Build history of the part. All positions in model axes, mm. Face numbers are marked on the shaded views. A direction names the side the tool comes from. Give positions to 0.01 mm unless a question says otherwise; leave off trailing zeros. Order: outer loops, then holes, each group sorted by start corner. A loop starts at its lowest first (then second) coordinate and runs counter-clockwise, first axis right, second up. Notation, with made-up numbers: (70, 1) - (98, 1) arc R29 cw to (98, 34) - close; hole circle Ø8 at (89, 20.25). An arc over 180 degrees is marked (long way). One line per item, written item: value.
```python
from build123d import *

# Parameters (mm, degrees)
F0_W        = 20
F0_H        = 50
F0_W_2      = 16
F0_H_2      = 46
F1_DEPTH    = 2
F2_DEPTH    = 36
F4_DEPTH    = 10
F5_R        = 1.875
F6_DEPTH    = 25
F7_T1_DEPTH = 2
F7_T3_DEPTH = 2
F7_T5_DEPTH = 61
F7_T7_DEPTH = 27
F7_T9_DEPTH = 75
F8_DEPTH    = 3
F9_DEPTH    = 3


# Not quite as in the source:
# - a fillet or chamfer that OpenCascade refuses, or shapes differently, is made with other operations: its cross-section is extruded or revolved along the edge and cut away or added


with BuildPart() as f1:
    # F0 (on Top) → F1 (new body)
    with BuildSketch(Plane.XY):
        Rectangle(F0_W, F0_H)
        Rectangle(F0_W_2, F0_H_2, mode=Mode.SUBTRACT)
        Rectangle(F0_W_2, F0_H_2)
    extrude(amount=F1_DEPTH)

    # F0 (on Top) → F2 (join)
    with BuildSketch(Plane.XY):
        Rectangle(F0_W, F0_H)
        Rectangle(F0_W_2, F0_H_2, mode=Mode.SUBTRACT)
    extrude(amount=F2_DEPTH)

    # F3 (on face) → F4 (join)
    with BuildSketch(Plane.XY.offset(36)):
        Polygon((10, -25), (10, 25), (8, 25), (8, 23), (8, -23), (8, -25), align=None)
    extrude(amount=F4_DEPTH)

    # F5 (on face) → F6 (cut)
    with BuildSketch(Plane(origin=(8, 0, 0), x_dir=(0, -1, 0), z_dir=(-1, 0, 0))):
        with Locations((15, 41)):
            Circle(F5_R)
        with Locations((-15, 41)):
            Circle(F5_R)
    extrude(amount=-F6_DEPTH, mode=Mode.SUBTRACT)

    # F7: fillet of radius 5 on 7 edges, made by hand

    # F7_s2 → F7_t1 (join)
    with BuildSketch(Plane.XZ.offset(23)):
        with BuildLine():
            ThreePointArc((8, 41), (6.5355339059, 37.4644660941), (3, 36))
            Line((3, 36), (8, 36))
            Line((8, 36), (8, 41))
        make_face()
    extrude(amount=F7_T1_DEPTH)

    # F7_s4 → F7_t3 (join)
    with BuildSketch(Plane.XZ.offset(-25)):
        with BuildLine():
            ThreePointArc((8, 41), (6.5355339059, 37.4644660941), (3, 36))
            Line((3, 36), (8, 36))
            Line((8, 36), (8, 41))
        make_face()
    extrude(amount=F7_T3_DEPTH)

    # F7_s6 → F7_t5 (cut)
    with BuildSketch(Plane.XY.offset(-12.5)):
        with BuildLine():
            ThreePointArc((-5, -25), (-8.5355339059, -23.5355339059), (-10, -20))
            Line((-10, -20), (-10, -25))
            Line((-10, -25), (-5, -25))
        make_face()
        with BuildLine():
            ThreePointArc((-5, 25), (-8.5355339059, 23.5355339059), (-10, 20))
            Line((-10, 20), (-10, 25))
            Line((-10, 25), (-5, 25))
        make_face()
    extrude(amount=F7_T5_DEPTH, mode=Mode.SUBTRACT)

    # F7_s8 → F7_t7 (cut)
    with BuildSketch(Plane.YZ.offset(-4.5)):
        with BuildLine():
            ThreePointArc((-25, 41), (-23.5355339059, 44.5355339059), (-20, 46))
            Line((-20, 46), (-25, 46))
            Line((-25, 46), (-25, 41))
        make_face()
        with BuildLine():
            ThreePointArc((25, 41), (23.5355339059, 44.5355339059), (20, 46))
            Line((20, 46), (25, 46))
            Line((25, 46), (25, 41))
        make_face()
    extrude(amount=F7_T7_DEPTH, mode=Mode.SUBTRACT)

    # F7_s10 → F7_t9 (cut)
    with BuildSketch(Plane.XZ.offset(-37.5)):
        with BuildLine():
            ThreePointArc((-10, 31), (-8.5355339059, 34.5355339059), (-5, 36))
            Line((-5, 36), (-10, 36))
            Line((-10, 36), (-10, 31))
        make_face()
    extrude(amount=F7_T9_DEPTH, mode=Mode.SUBTRACT)

    # F8 (add): a face of the model
    f8_faces = [f1.faces().sort_by_distance(p)[0] for p in [
        (10, 0, 22.721056124),
    ]]
    extrude(f8_faces, amount=F8_DEPTH)

    # F5 (on face) → F9 (cut)
    with BuildSketch(Plane(origin=(8, 0, 0), x_dir=(0, -1, 0), z_dir=(-1, 0, 0))):
        with BuildLine():
            ThreePointArc((-9.25, 41), (-10.0306257188, 43.8927183155), (-12.1605458271, 46))
            Line((-12.1605458271, 46), (-17.8394541729, 46))
            ThreePointArc((-17.8394541729, 46), (-17.8927183155, 36.0306257188), (-9.25, 41))
        make_face()
        with Locations((-15, 41)):
            Circle(F5_R, mode=Mode.SUBTRACT)
        with BuildLine():
            ThreePointArc((12.1605458271, 46), (12.1072816845, 36.0306257188), (20.75, 41))
            ThreePointArc((20.75, 41), (19.9693742812, 43.8927183155), (17.8394541729, 46))
            Line((17.8394541729, 46), (12.1605458271, 46))
        make_face()
        with Locations((15, 41)):
            Circle(F5_R, mode=Mode.SUBTRACT)
    extrude(amount=-F9_DEPTH, mode=Mode.SUBTRACT)


solid = f1.part
```
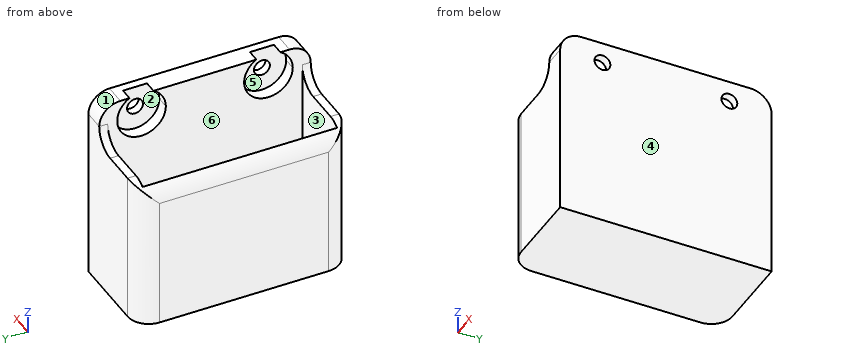
(1) 3-axis set-ups, long thin cutter, end or side, ignore diameter. For the marked faces 1 and 2: which of +Z, -Z, +X, -X, +Y, -Y reach the whole face in a straight line?
Completed:
face 1: +Z, +X, -X, +Y
face 2: -X
(2) Pull direction X, two halves, no side cores. Call the marked faces 3, 4, 5 and 6: +X half, -X half, draft (parallel to the pull), parting line (faces both ways), or undercut.
Completed:
face 3: undercut
face 4: +X half
face 5: -X half
face 6: undercut
(3) Slice it at A-A, the plane y = 15. Give the cut face in (x, z) (3 decimals).
Completed:
outline: (-10, 0) - (13, 0) - (13, 39.125) - (11, 39.125) - (11, 35.25) - (8, 35.25) - (8, 2) - (-8, 2) - (-8, 35) arc R5 ccw to (-10, 31) - close; (11, 42.875) - (13, 42.875) - (13, 46) - (11, 46) - close
(4) Slice it at B-B, the plane x = 2.25. Give the cut face in (y, z).
Completed:
outline: (-25, 0) - (25, 0) - (25, 36) - (23, 36) - (23, 2) - (-23, 2) - (-23, 36) - (-25, 36) - close
(5) Slice it at D-D, the plane y = -2. Give the cut face in (x, z), and give its area (3 significant figures).
Completed:
outline: (-10, 0) - (13, 0) - (13, 46) - (8, 46) - (8, 2) - (-8, 2) - (-8, 35) arc R5 ccw to (-10, 31) - close
area: 330 mm²
(6) Drill centre lines: line 1 (Y direction, x = 9, z = 41); line 2 (Z direction, x = 11.8, y = -15) (3 decimals); line 3 (Y direction, x = -2, z = 7). Where is each one in solid material? Low to high.
Completed:
line 1: -25 to -20.75, -9.25 to 9.25, 20.75 to 25
line 2: 0 to 39.125, 42.875 to 46
line 3: -25 to -23, 23 to 25
(7) Pin check, flat tips, straight feed: P1, Ø2, axis at x = 0, y = 24, coming from the +Z side; P2, Ø12, axis at y = 14, z = 40.5, coming from the -X side; P3, Ø8.5, axis at y = -12, z = 43, coming from the -X side. Stop position of each tip, or through.
Completed:
P1: z = 36
P2: x = -8.57
P3: x = 8
(8) Slice it at C-C, the plane z = 26.5. Give the cut face in (x, y).
Completed:
outline: (-10, -20) arc R5 ccw to (-5, -25) - (13, -25) - (13, 25) - (-5, 25) arc R5 ccw to (-10, 20) - close; hole (-8, -23) - (8, -23) - (8, 23) - (-8, 23) - close
